The listing builds one solid part. Answer for the finished solid, in the listing's coordinates (mm). Coordinates: 2 decimals unless noted, no trailing zeros. Order: outer loops, then holes, each group sorted by start corner. A loop starts at its lowest first (then second) coordinate and runs counter-clockwise, first axis right, second up. Notation, with made-up numbers: (88, -34.75) -> (105, -34.75) arc R25 ccw to (105, -9.75) -> close; hole circle Ø3 at (83, 57). An arc over 180 degrees is marked (long way). Return JSON: item names as keys, results as strings.
from build123d import *

# Parameters (mm, degrees)
F0_R     = 12.7
F1_DEPTH = 6.35


# Not quite as in the source:
# - a feature names something its author has since deleted; it is built from what else it names


with BuildPart() as f1:
    # F0 (on Front) → F1 (new body)
    with BuildSketch(Plane.XZ):
        with BuildLine():
            ThreePointArc((16.4814082308, 37.1287725662), (16.4903338535, 37.6145443772), (16.51, 38.1))
            ThreePointArc((16.51, 38.1), (0, 54.61), (-16.51, 38.1))
            ThreePointArc((-16.51, 38.1), (-0.4858240981, 21.5971494903), (16.4814082308, 37.1287725662))
        make_face()
        with Locations((0, 38.1)):
            Circle(F0_R, mode=Mode.SUBTRACT)
        with BuildLine():
            ThreePointArc((16.4814082308, 37.1287725662), (-0.4858240981, 21.5971494903), (-16.51, 38.1))
            ThreePointArc((-16.51, 38.1), (-24.8582581267, 22.5634685942), (-41.3111088486, 16.2088698662))
            ThreePointArc((-41.3111088486, 16.2088698662), (-31.7141609442, 10.5061174344), (-27.94, 0))
            ThreePointArc((-27.94, 0), (-32.0196049569, -10.8657893902), (-42.2422869864, -16.3617267808))
            ThreePointArc((-42.2422869864, -16.3617267808), (-25.2542323654, -22.3516257894), (-16.51, -38.1))
            ThreePointArc((-16.51, -38.1), (0, -21.59), (16.51, -38.1))
            ThreePointArc((16.51, -38.1), (25.2542323654, -22.3516257894), (42.2422869864, -16.3617267808))
            ThreePointArc((42.2422869864, -16.3617267808), (28.118646251, -2.4221859395), (37.5884063644, 15.0166118942))
            ThreePointArc((37.5884063644, 15.0166118942), (22.5582227264, 21.7995063444), (16.4814082308, 37.1287725662))
        make_face()
        Circle(F0_R, mode=Mode.SUBTRACT)
        with BuildLine():
            ThreePointArc((-27.94, 0), (-31.7141609442, 10.5061174344), (-41.3111088486, 16.2088698662))
            ThreePointArc((-41.3111088486, 16.2088698662), (-43.3621139683, 16.2630178255), (-45.4020575599, 16.4825266996))
            ThreePointArc((-45.4020575599, 16.4825266996), (-60.9531302457, -0.4762269364), (-44.45, -16.51))
            ThreePointArc((-44.45, -16.51), (-43.3477588373, -16.4118117369), (-42.2422869864, -16.3617267808))
            ThreePointArc((-42.2422869864, -16.3617267808), (-32.0196049569, -10.8657893902), (-27.94, 0))
        make_face()
        with Locations((-44.45, 0)):
            Circle(F0_R, mode=Mode.SUBTRACT)
        with BuildLine():
            ThreePointArc((46.209319854, 16.4159950552), (41.9691064238, 15.2835688562), (37.5884063644, 15.0166118942))
            ThreePointArc((37.5884063644, 15.0166118942), (28.118646251, -2.4221859395), (42.2422869864, -16.3617267808))
            ThreePointArc((42.2422869864, -16.3617267808), (43.3477588373, -16.4118117369), (44.45, -16.51))
            ThreePointArc((44.45, -16.51), (56.1243329574, -11.6743329574), (60.96, 0))
            ThreePointArc((60.96, 0), (56.7306040322, 11.0348024271), (46.209319854, 16.4159950552))
        make_face()
        with BuildLine():
            ThreePointArc((46.9166774243, 12.4581500426), (43.685710075, -12.6769815378), (43.4979424401, 12.6642641477))
            ThreePointArc((43.4979424401, 12.6642641477), (43.8445127875, 12.3613055932), (44.1938141149, 12.0614998657))
            ThreePointArc((44.1938141149, 12.0614998657), (45.5606208941, 12.2229266237), (46.9166774243, 12.4581500426))
        make_face(mode=Mode.SUBTRACT)
        with BuildLine():
            ThreePointArc((-16.51, -38.1), (0, -54.61), (16.51, -38.1))
            ThreePointArc((16.51, -38.1), (0, -21.59), (-16.51, -38.1))
        make_face()
        with Locations((0, -38.1)):
            Circle(F0_R, mode=Mode.SUBTRACT)
    extrude(amount=F1_DEPTH)


solid = f1.part
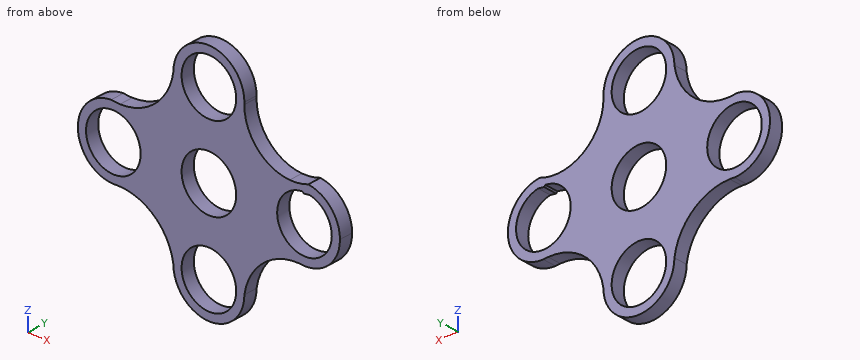
1. The part is cut by section A-A on x = 0. Give the vertices of the cut face in (y, z), and give its area (3 significant figures).
Answer block:
{"outline": "(-6.35, -54.61) -> (0, -54.61) -> (0, -50.8) -> (-6.35, -50.8) -> close; (-6.35, -25.4) -> (0, -25.4) -> (0, -12.7) -> (-6.35, -12.7) -> close; (-6.35, 12.7) -> (0, 12.7) -> (0, 25.4) -> (-6.35, 25.4) -> close; (-6.35, 50.8) -> (0, 50.8) -> (0, 54.61) -> (-6.35, 54.61) -> close", "area": "210 mm2"}
2. Consider line 1 (Z direction, x = 0, y = -3.75); line 2 (X direction, y = -2.25, z = 38); line 3 (Z direction, x = 4.5, y = -5.25). Determine where each line is inside the solid, lowest interval first. Write a range as from..to.
Answer block:
{"line 1": "z = -54.61..-50.8, -25.4..-12.7, 12.7..25.4, 50.8..54.61", "line 2": "x = -16.52..-12.7, 12.7..16.51", "line 3": "z = -53.98..-49.98, -26.22..-11.88, 11.88..26.22, 49.98..53.98"}
3. Each of these flat-tipped pins is pushed along its axis until it touches: pin 1 Ø1.5 at (x, z) = (-28.5, -8.5) entering from +Y; pin 2 Ø23 at (x, z) = (44.45, 0) entering from +Y; pin 3 Ø2 at (x, y) = (-41, -1.5) entering from +Z. Where does it stop, or does it pass through?
Answer block:
{"pin 1": "stops at y = 0", "pin 2": "passes through", "pin 3": "stops at z = 16.26"}
4. The part is cut by section D-D on z = 9.5. Give the vertices of the cut face in (x, y), and give its area (3 significant figures).
Answer block:
{"outline": "(-57.95, -6.35) -> (-52.88, -6.35) -> (-52.88, 0) -> (-57.95, 0) -> close; (-36.02, -6.35) -> (-8.43, -6.35) -> (-8.43, 0) -> (-36.02, 0) -> close; (8.43, -6.35) -> (36.02, -6.35) -> (36.02, 0) -> (8.43, 0) -> close; (52.88, -6.35) -> (57.95, -6.35) -> (57.95, 0) -> (52.88, 0) -> close", "area": "415 mm2"}
5. The part is cut by section B-B on y = -4.25. Give the vertices of the cut face in (x, z), and give its area (3 significant figures).
Answer block:
{"outline": "(-45.4, 16.48) arc R16.51 ccw to (-44.45, -16.51) arc R25.4 cw to (-16.51, -38.1) arc R16.51 ccw to (16.51, -38.1) arc R25.4 cw to (44.45, -16.51) arc R16.51 ccw to (46.21, 16.42) arc R21.97 cw to (16.51, 38.1) arc R16.51 ccw to (-16.51, 38.1) arc R25.4 cw to start; hole circle Ø25.4 at (-44.45, 0); hole circle Ø25.4 at (0, -38.1); hole circle Ø25.4 at (0, 0); hole circle Ø25.4 at (0, 38.1); hole (43.5, 12.66) arc R12.7 ccw (long way) to (46.92, 12.46) arc R25.4 cw to (44.19, 12.06) arc R50.8 cw to start", "area": "3,980 mm2"}
6. The part is cut by section C-C on z = -33. Give the vertices of the cut face in (x, y), and give its area (3 significant figures).
Answer block:
{"outline": "(-17.8, -6.35) -> (-11.63, -6.35) -> (-11.63, 0) -> (-17.8, 0) -> close; (11.63, -6.35) -> (17.8, -6.35) -> (17.8, 0) -> (11.63, 0) -> close", "area": "78.4 mm2"}
